Could you check a few things on this drawing? It's one solid part, dimensions in mm from its lowest x, y, z. Give positions to 0.01 mm unless a question says otherwise; leave off trailing zeros. Loops run counter-clockwise (first coordinate to the right, second up) from the corner with the lowest first, then second, coordinate; pieces in that order, holes last. Notation, with made-up numbers: (40, 74.5) - (91, 74.5) arc R15 ccw to (91, 97.5) - close; hole circle Ø7 at (45, 37). An arc over 180 degrees is marked (long way). Return JSON: item names as keys, results as strings. Group by question number.
(1) If we section it at C-C (y = 54): Please give me the cut outline in (x, z) (1 decimal).
(2) If we section it at B-B (z = 27): State how many separate pieces and enclosed holes the cut face has.
(3) If we section it at D-D (x = 88.5): Please give me the cut outline in (y, z).
(4) I need wall thicknesses on probe 1 along X at (y, z) = (35, 27.5) (1 decimal); probe 2 along X at (y, z) = (26, 18.5) (1 decimal); probe 3 along Y at (x, z) = (70, 25.5) (1 decimal). Which ranges of each line are inside material? Lowest first, please. Write a range as [from, to].
(5) For P1, Ø6, axis at y = 41.5, z = 11.5, coming from the -X side; P2, Ø1.5, axis at x = 66.5, z = 12, coming from the +Y side; P3, Ø5, axis at x = 71.06, y = 29.88, coming from the +Z side; P4, Ø5, axis at x = 96.5, z = 21.5, coming from the -Y side, each with a flat end and sliding along its axis, tell me the tip position at first contact or that it passes through.
(6) If we section it at A-A (x = 72.5): Please give me the cut outline in (y, z), then the cut area to 3 significant figures.
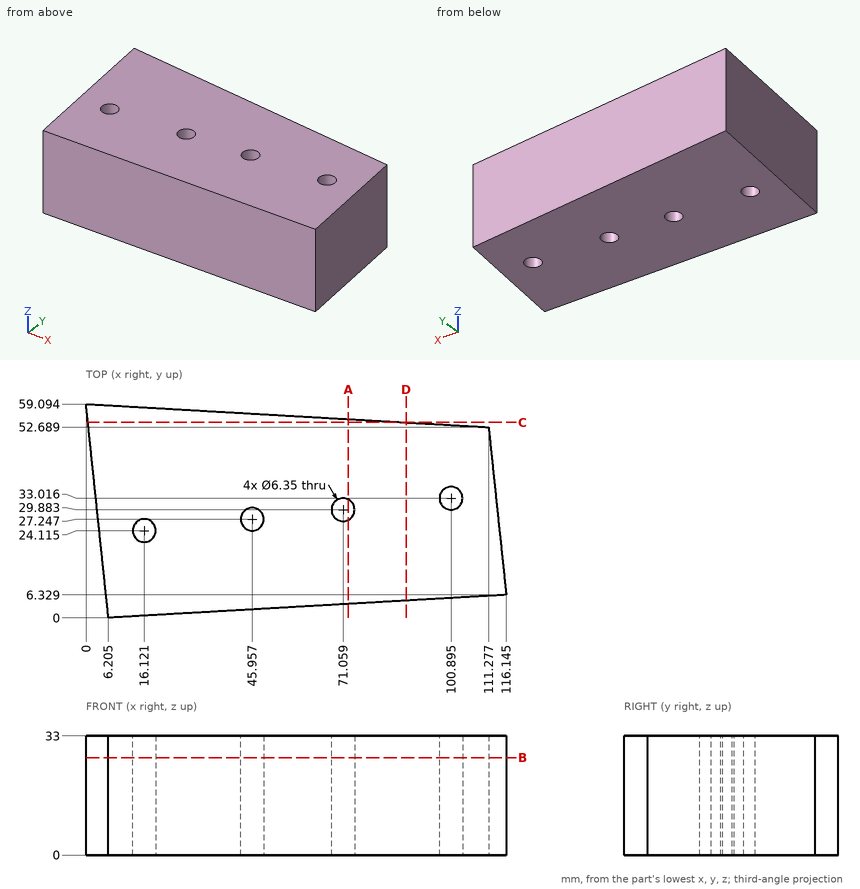
Values:
{
 "1": {"outline": "(0.5, 0) - (88.5, 0) - (88.5, 33) - (0.5, 33) - close"},
 "2": {"separate pieces": "1", "enclosed holes": "4"},
 "3": {"outline": "(4.74, 0) - (54, 0) - (54, 33) - (4.74, 33) - close"},
 "4": {"probe 1": "[2.5, 98.4], [103.4, 113.1]", "probe 2": "[3.5, 13.6], [18.7, 43], [48.9, 114.1]", "probe 3": "[3.7, 26.9], [32.9, 55.1]"},
 "5": {"P1": "x = 1.53", "P2": "y = 55.31", "P3": "through", "P4": "y = 5.05"},
 "6": {"outline": "(3.82, 0) - (27.05, 0) - (27.05, 33) - (3.82, 33) - close; (32.71, 0) - (54.92, 0) - (54.92, 33) - (32.71, 33) - close", "area": "1,500 mm2"}
}
